The listing builds one solid part. Answer for the finished solid, in the listing's coordinates (mm). A direction names the side the tool comes from. Coordinates: 2 decimals unless noted, no trailing zeros. Write each loop counter-clockwise with the first axis right and the second up, starting at its lowest first coordinate (ties: lowest second). Pieces come first, ordered by that corner, then holes.
from build123d import *

# Parameters (mm, degrees)
F1_DEPTH = 16
F2_R     = 10
F3_DEPTH = 25
F4_W     = 60
F4_H     = 8
F5_DEPTH = 25
F7_DEPTH = 5


with BuildPart() as f1:
    # F0 (on Top) → F1 (new body)
    with BuildSketch(Plane.XY):
        with BuildLine():
            Line((75, -5), (75, 0))
            Line((75, 0), (75, 5))
            ThreePointArc((75, 5), (73.535534, 8.535534), (70, 10))
            Line((70, 10), (0, 10))
            ThreePointArc((0, 10), (-27.620499, 0), (0, -10))
            Line((0, -10), (70, -10))
            ThreePointArc((70, -10), (73.535534, -8.535534), (75, -5))
        make_face()
    extrude(amount=F1_DEPTH)

    # F2 (on face) → F3 (cut)
    with BuildSketch(Plane.XY.offset(16)):
        with Locations((-12, 0)):
            Circle(F2_R)
    extrude(amount=-F3_DEPTH, mode=Mode.SUBTRACT)

    # F4 (on face) → F5 (cut)
    with BuildSketch(Plane.XZ.offset(10)):
        with Locations((35, 8)):
            Rectangle(F4_W, F4_H)
    extrude(amount=-F5_DEPTH, mode=Mode.SUBTRACT)

    # F6 (on face) → F7 (cut)
    with BuildSketch(Plane.XY.offset(16)):
        with BuildLine():
            ThreePointArc((-10.00009, 15.491945), (-12.000217, 15.620499), (-14.000341, 15.491889))
            Line((-14.000341, 15.491889), (-14.000341, 9.797889))
            ThreePointArc((-14.000341, 9.797889), (-12.00022, 10), (-10.00009, 9.797977))
            Line((-10.00009, 9.797977), (-10.00009, 15.491945))
        make_face()
        with BuildLine():
            Line((-14.000341, -9.797889), (-14.000341, -15.491889))
            ThreePointArc((-14.000341, -15.491889), (-12.000344, -15.620499), (-10.000341, -15.491977))
            Line((-10.000341, -15.491977), (-10.00009, -9.797977))
            ThreePointArc((-10.00009, -9.797977), (-12.00022, -10), (-14.000341, -9.797889))
        make_face()
    extrude(amount=-F7_DEPTH, mode=Mode.SUBTRACT)


solid = f1.part
Q1. The part is cut by section A-A, the plane y = 0. Write down the section's boundary in (x, z).
Answers below:
outline: (-27.62, 0) - (-22, 0) - (-22, 16) - (-27.62, 16) - close; (-2, 0) - (75, 0) - (75, 16) - (-2, 16) - close; hole (5, 4) - (65, 4) - (65, 12) - (5, 12) - close
Q2. Given pin 1 (5.5 mm diameter, centred on y = -11.5, z = 12.5, fed in from +X); pin 2 (1 mm diameter, centred on x = 56.5, z = 5.5, fed in from -Y); pin 3 (8 mm diameter, centred on x = 30, z = 11, fed in from -Y); pin 4 (1.5 mm diameter, centred on y = 13, z = 13, fed in from -X), each flat-ended and moving along its own axis, determine where each tip first touches the part or whether it passes through.
Answers below:
pin 1: stops at x = 73.31
pin 2: passes through
pin 3: stops at y = -10
pin 4: stops at x = -21.69
Q3. The part is cut by section D-D, the plane z = 14. Write down the section's boundary in (x, y), then the cut area to 3 significant figures.
Answers below:
outline: (-14, -15.49) - (-14, -9.8) arc R10 cw to (-14, 9.8) - (-14, 15.49) arc R15.62 ccw to start; (-10, -15.49) arc R15.62 ccw to (0, -10) - (70, -10) arc R5 ccw to (75, -5) - (75, 5) arc R5 ccw to (70, 10) - (0, 10) arc R15.62 ccw to (-10, 15.49) - (-10, 9.8) arc R10 cw to (-10, -9.8) - close
area: 1,850 mm2
Q4. The part is cut by section B-B, the plane z = 7.5. Write down the section's boundary in (x, y).
Answers below:
outline: (0, -10) - (5, -10) - (5, 10) - (0, 10) arc R15.62 ccw (long way) to start; (65, -10) - (70, -10) arc R5 ccw to (75, -5) - (75, 5) arc R5 ccw to (70, 10) - (65, 10) - close; hole circle Ø20 at (-12, 0)
Q5. The part is cut by section C-C, the plane x = -12. Write down the section's boundary in (y, z), then the cut area to 3 significant figures.
Answers below:
outline: (-15.62, 0) - (-10, 0) - (-10, 11) - (-15.62, 11) - close; (10, 0) - (15.62, 0) - (15.62, 11) - (10, 11) - close
area: 124 mm2
Q6. Which of the six approach directions +Z, -Z, +X, -X, +Y, -Y give full straight-line access (tool end or side, diameter ignored) to faces 4 (the face through (35, -10, 13)), 5 (the face through (35, 10, 13)), 6 (the face through (-12, 13, 11))?
Answers below:
face 4: +Z, -Z, +X, -Y
face 5: +Z, -Z, +X, +Y
face 6: +Z, +Y, -Y
Q7. Find the intervals of material crossed by probe 1 along Z at (x, y) = (37.5, -7); probe 2 along Y at (x, z) = (-12, 5); probe 3 along Y at (x, z) = (-14, 2.5), in increasing order.
Answers below:
probe 1: z = 0 to 4, 12 to 16
probe 2: y = -15.62 to -10, 10 to 15.62
probe 3: y = -15.49 to -9.8, 9.8 to 15.49
Q8. Determine the mould class of faces 1 (the face through (-22.4, 0.2, 16)), 2 (the face through (35, 0, 4)), 3 (the face through (73, -9, 8)) for opening direction Z: released by +Z, released by -Z, zero draft, split by the parting line, or undercut.
Answers below:
face 1: released by +Z
face 2: undercut
face 3: zero draft
